Input: part model. Units: mm. Frame: model coordinates. A direction names the side the tool comes from. Coordinates: 2 decimals unless noted, no trailing zeros. Write each loop counter-clockwise with the first axis right and the second up, starting at its lowest first coordinate (ties: lowest second). Pieces come first, ordered by that corner, then holes. Notation, with made-up numbers: (87.25, 36.5) - (123.25, 36.5) arc R35 cw to (123.25, 69.5) - close; hole circle Ø9 at (-36, 65.5). An arc over 180 degrees is marked (long way). Use a Markdown table: item, result. Add a question column.
Q1. Mould query, pull axis Y, two halves, no side actions, for faces 1 (the face through (-44.702, -19.906, 67.455)), 2 (the face through (-44, 0, 35)), 3 (the face through (-21, -5, 67)). Classes: released by +Y, released by -Y, zero draft, split by the parting line, or undercut.
Q2. Section query A-A (z = 61). Return the cut outline in (x, y), then the cut area to 3 significant figures.
Q3. Section query C-C (y = 3). Return the cut outline in (x, z).
Q4. Material intervals for probe 1 along Y at (x, z) = (-30, 40.5); probe 2 along Y at (x, z) = (-5, 40.5); probe 3 along Z at (x, y) = (-60.5, -3), sorted ascending. Write a range as from..to.
Q5. Pin query (flat end, axial travel): P1, Ø5, axis at x = -13, z = 72, coming from the -Y side; P2, Ø12, axis at x = -72.5, y = -28.5, coming from the +Z side; P3, Ø4, axis at y = -47.5, z = 50, coming from the +X side. Return the tip coordinate at first contact, or that it passes through.
Q6. Section query B-B (x = -13). Return the cut outline in (y, z), then the cut area to 3 significant figures.
Q7. Set-up query: faces 4 (the face through (-75, -18, 65)), 5 (the face through (-85, -5, 51)), 6 (the face through (-20, 7, 48)). Return all of +Z, -Z, +X, -X, +Y, -Y with unobstructed straight access to the full face (end or side cutting, diameter ignored); none if empty.
Q8. Section query D-D (x = -30.5). Return the cut outline in (y, z).
from build123d import *

# Parameters (mm, degrees)
BOSS_EXTRUDE1_DEPTH            = 60
SKETCH2_W                      = 30
SKETCH2_H                      = 10
CUT_EXTRUDE1_DEPTH             = 253
BOSS_EXTRUDE2_DEPTH            = 15
CUT_EXTRUDE5_DEPTH             = 10
SKETCH8_R                      = 5
CUT_EXTRUDE6_DEPTH             = 124
BOSS_EXTRUDE3_DEPTH            = 15
SKETCH15_W                     = 45
SKETCH15_H                     = 60
CUT_EXTRUDE8_DEPTH             = 90
BOSS_EXTRUDE4_DEPTH            = 10
F_1_2_1_2_DIAMETER_HOLE7_D     = 5
F_1_2_1_2_DIAMETER_HOLE7_DEPTH = 10
F_1_2_1_2_DIAMETER_HOLE7_TIP   = 1.357389249
F_10_0_10_DIAMETER_HOLE4_D     = 10
F_10_0_10_DIAMETER_HOLE4_DEPTH = 20
F_10_0_10_DIAMETER_HOLE4_TIP   = 2.714778498


with BuildPart() as part:
    # Sketch1 → Boss-Extrude1 (new body)
    with BuildSketch(Plane.XY):
        with BuildLine():
            Line((-90, 0), (-90, 5))
            ThreePointArc((-90, 5), (-88.535533906, 8.535533906), (-85, 10))
            Line((-85, 10), (-70, 10))
            Line((-70, 10), (-70, 5))
            Line((-70, 5), (-20, 5))
            Line((-20, 5), (-20, 10))
            Line((-20, 10), (-5, 10))
            ThreePointArc((-5, 10), (-1.464466094, 8.535533906), (0, 5))
            Line((0, 5), (0, 0))
            Line((0, 0), (-10, -10))
            Line((-10, -10), (-10, -30))
            Line((-10, -30), (0, -40))
            Line((0, -40), (0, -45))
            ThreePointArc((0, -45), (-1.464466094, -48.535533906), (-5, -50))
            Line((-5, -50), (-20, -50))
            Line((-20, -50), (-20, -45))
            Line((-20, -45), (-70, -45))
            Line((-70, -45), (-70, -50))
            Line((-70, -50), (-85, -50))
            ThreePointArc((-85, -50), (-88.535533906, -48.535533906), (-90, -45))
            Line((-90, -45), (-90, -40))
            Line((-90, -40), (-80, -30))
            Line((-80, -30), (-80, -10))
            Line((-80, -10), (-90, 0))
        make_face()
    extrude(amount=BOSS_EXTRUDE1_DEPTH)

    # Sketch2 → Cut-Extrude1 (cut)
    with BuildSketch(Plane(origin=(0, 0, 0), x_dir=(0, 0, -1), z_dir=(1, 0, 0))):
        with Locations((-30, -45)):
            Rectangle(SKETCH2_W, SKETCH2_H)
    extrude(amount=-CUT_EXTRUDE1_DEPTH, mode=Mode.SUBTRACT)

    # Sketch3 → Boss-Extrude2 (add)
    with BuildSketch(Plane.XY.offset(60)):
        with BuildLine():
            Line((-85, -5), (-80, -10))
            Line((-80, -10), (-80, -30))
            Line((-80, -30), (-85, -35))
            Line((-85, -35), (-52.5, -35))
            ThreePointArc((-52.5, -35), (-45, -27.5), (-37.5, -35))
            Line((-37.5, -35), (-5, -35))
            Line((-5, -35), (-10, -30))
            Line((-10, -30), (-10, -10))
            Line((-10, -10), (-5, -5))
            Line((-5, -5), (-37.5, -5))
            ThreePointArc((-37.5, -5), (-45, -12.5), (-52.5, -5))
            Line((-52.5, -5), (-85, -5))
        make_face()
    extrude(amount=BOSS_EXTRUDE2_DEPTH)

    # Sketch4 → Cut-Extrude5 (cut)
    with BuildSketch(Plane.XY.offset(75)):
        with BuildLine():
            Line((-80, -12.5), (-70, -12.5))
            ThreePointArc((-70, -12.5), (-62.5, -20), (-70, -27.5))
            Line((-70, -27.5), (-80, -27.5))
            Line((-80, -27.5), (-80, -12.5))
        make_face()
        with BuildLine():
            Line((-10, -12.5), (-10, -27.5))
            Line((-10, -27.5), (-20, -27.5))
            ThreePointArc((-20, -27.5), (-27.5, -20), (-20, -12.5))
            Line((-20, -12.5), (-10, -12.5))
        make_face()
    extrude(amount=-CUT_EXTRUDE5_DEPTH, mode=Mode.SUBTRACT)

    # Sketch8 → Cut-Extrude6 (cut)
    with BuildSketch(Plane.XY.offset(65)):
        with Locations((-20, -20)):
            Circle(SKETCH8_R)
        with Locations((-70, -20)):
            Circle(SKETCH8_R)
    extrude(amount=-CUT_EXTRUDE6_DEPTH, mode=Mode.SUBTRACT)

    # Sketch11 → Boss-Extrude3 (add)
    with BuildSketch(Plane.XY.offset(75)):
        with BuildLine():
            ThreePointArc((-51.236095645, -9.166666667), (-57.5, -20), (-51.236095645, -30.833333333))
            ThreePointArc((-51.236095645, -30.833333333), (-45, -27.5), (-38.763904355, -30.833333333))
            ThreePointArc((-38.763904355, -30.833333333), (-32.5, -20), (-38.763904355, -9.166666667))
            ThreePointArc((-38.763904355, -9.166666667), (-45, -12.5), (-51.236095645, -9.166666667))
        make_face()
    extrude(amount=BOSS_EXTRUDE3_DEPTH)

    # Sketch15 → Cut-Extrude8 (cut, symmetric)
    with BuildSketch(Plane.ZY.offset(80)):
        with Locations((22.5, -20)):
            Rectangle(SKETCH15_W, SKETCH15_H)
    extrude(amount=CUT_EXTRUDE8_DEPTH, both=True, mode=Mode.SUBTRACT)

    # Sketch16 → Boss-Extrude4 (add)
    with BuildSketch(Plane(origin=(0, 0, 45), x_dir=(-1, 0, 0), z_dir=(0, 0, -1))):
        with BuildLine():
            Line((10, -10), (80, -10))
            Line((80, -10), (90, 0))
            Line((90, 0), (90, 5))
            ThreePointArc((90, 5), (88.535533906, 8.535533906), (85, 10))
            Line((85, 10), (70, 10))
            Line((70, 10), (70, 5))
            Line((70, 5), (20, 5))
            Line((20, 5), (20, 10))
            Line((20, 10), (5, 10))
            ThreePointArc((5, 10), (1.464466094, 8.535533906), (0, 5))
            Line((0, 5), (0, 0))
            Line((0, 0), (10, -10))
        make_face()
        with BuildLine():
            Line((80, -30), (10, -30))
            Line((10, -30), (0, -40))
            Line((0, -40), (0, -45))
            ThreePointArc((0, -45), (1.464466094, -48.535533906), (5, -50))
            Line((5, -50), (20, -50))
            Line((20, -50), (20, -45))
            Line((20, -45), (70, -45))
            Line((70, -45), (70, -50))
            Line((70, -50), (85, -50))
            ThreePointArc((85, -50), (88.535533906, -48.535533906), (90, -45))
            Line((90, -45), (90, -40))
            Line((90, -40), (80, -30))
        make_face()
    extrude(amount=BOSS_EXTRUDE4_DEPTH)

    # Ø1.2 (1.2) Diameter Hole7
    with Locations(Plane(origin=(-45.096109005, -2.501848071, 60), x_dir=(1, 0, 0), z_dir=(0, 0, 1))):
        with Locations((0, 0), (0, -34.996303858)):
            Hole(F_1_2_1_2_DIAMETER_HOLE7_D / 2, depth=F_1_2_1_2_DIAMETER_HOLE7_DEPTH)
            with Locations((0, 0, -(F_1_2_1_2_DIAMETER_HOLE7_DEPTH + F_1_2_1_2_DIAMETER_HOLE7_TIP / 2))):  # 123° drill point
                Cone(0, F_1_2_1_2_DIAMETER_HOLE7_D / 2, F_1_2_1_2_DIAMETER_HOLE7_TIP, mode=Mode.SUBTRACT)

    # Ø10.0 (10) Diameter Hole4
    with Locations(Plane(origin=(-45, -20, 90), x_dir=(1, 0, 0), z_dir=(0, 0, 1))):
        with Locations((0, 0)):
            Hole(F_10_0_10_DIAMETER_HOLE4_D / 2, depth=F_10_0_10_DIAMETER_HOLE4_DEPTH)
            with Locations((0, 0, -(F_10_0_10_DIAMETER_HOLE4_DEPTH + F_10_0_10_DIAMETER_HOLE4_TIP / 2))):  # 123° drill point
                Cone(0, F_10_0_10_DIAMETER_HOLE4_D / 2, F_10_0_10_DIAMETER_HOLE4_TIP, mode=Mode.SUBTRACT)


solid = part.part
Values follow:
| question | item | result |
|---|---|---|
| 1 | face 1 | undercut |
| 1 | face 2 | zero draft |
| 1 | face 3 | released by +Y |
| 2 | outline | (-85, -35) - (-52.5, -35) arc R7.5 cw to (-37.5, -35) - (-5, -35) - (-10, -30) - (-10, -10) - (-5, -5) - (-37.5, -5) arc R7.5 cw to (-52.5, -5) - (-85, -5) - (-80, -10) - (-80, -30) - close; hole circle Ø10 at (-70, -20); hole circle Ø10 at (-20, -20) |
| 2 | area | 1,820 mm2 |
| 3 | outline | (-90, 35) - (0, 35) - (0, 60) - (-90, 60) - close |
| 4 | probe 1 | -45..-30, -10..5 |
| 4 | probe 2 | -50..-35, -5..10 |
| 4 | probe 3 | 35..60 |
| 5 | P1 | y = -35 |
| 5 | P2 | z = 75 |
| 5 | P3 | x = -0.03 |
| 6 | outline | (-50, 35) - (-30, 35) - (-30, 45) - (-10, 45) - (-10, 35) - (10, 35) - (10, 60) - (-5, 60) - (-5, 75) - (-12.5, 75) - (-12.5, 65) - (-27.5, 65) - (-27.5, 75) - (-35, 75) - (-35, 60) - (-50, 60) - close |
| 6 | area | 1,600 mm2 |
| 7 | face 4 | +Z, -X |
| 7 | face 5 | +Z, -Z, -X |
| 7 | face 6 | +Z, -Z, +Y |
| 8 | outline | (-45, 35) - (-30, 35) - (-30, 45) - (-10, 45) - (-10, 35) - (5, 35) - (5, 60) - (-5, 60) - (-5, 75) - (-35, 75) - (-35, 60) - (-45, 60) - close |
